Could you check a few things on this drawing? It's one solid part, dimensions in mm from its lowest x, y, z. A direction names the side the tool comes from. Round coordinates to 2 decimals unless told otherwise and drop trailing zeros. Write each loop counter-clockwise with the first axis right and the second up, starting at its lowest first coordinate (ties: lowest second). Pieces come first, ordered by that corner, then holes. Notation, with made-up numbers: (-34.5, 80.5) -> (14.5, 80.5) arc R15 cw to (14.5, 96.5) -> close; hole circle Ø6 at (39.25, -39.75). An arc over 180 degrees is marked (long way). Answer in a Markdown table with one row per item.
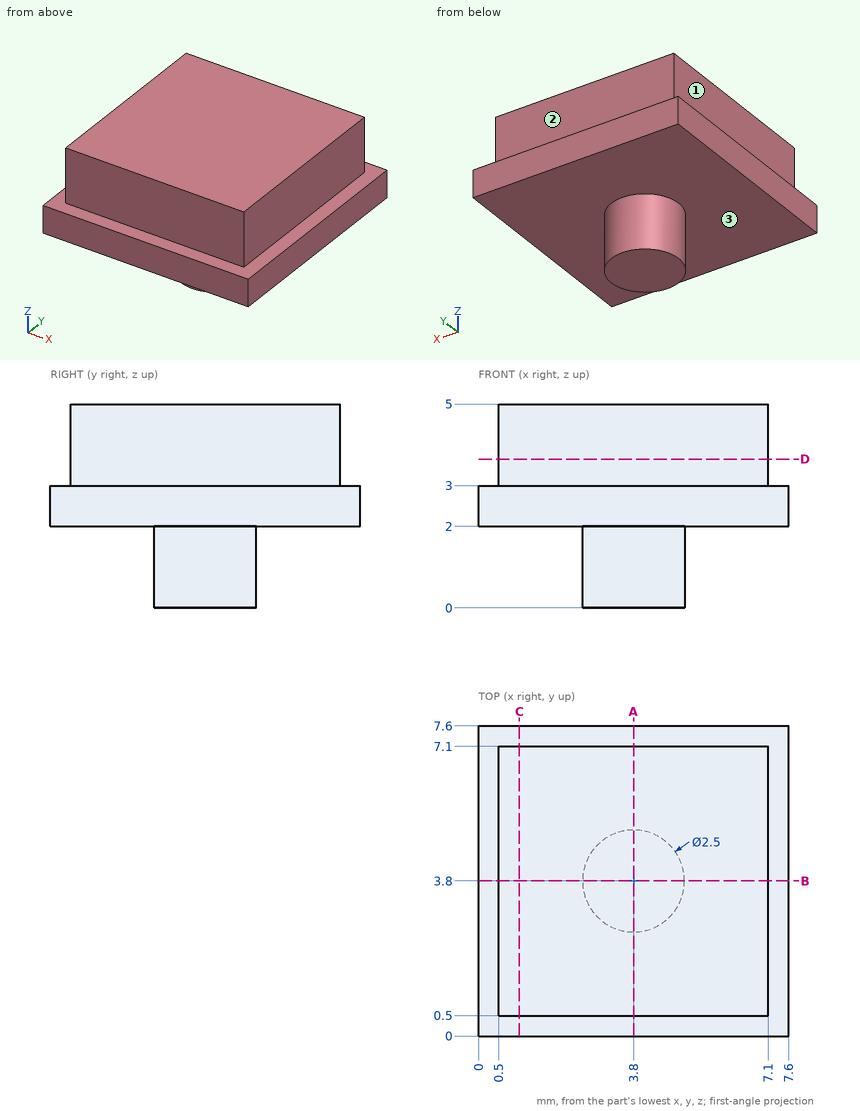
1) For pin 1 (1.6 mm diameter, centred on y = 2.5, z = 4, fed in from +X); pin 2 (3 mm diameter, centred on x = 1.5, z = 1.5, fed in from +Y); pin 3 (1 mm diameter, centred on x = 4, z = 4, fed in from -Y); pin 4 (1 mm diameter, centred on x = 4.5, y = 6.5, fed in from -Z), each with a flat end and sliding along its axis, tell me the tip position at first contact or that it passes through.
Findings:
| item | result |
|---|---|
| pin 1 | stops at x = 7.1 |
| pin 2 | stops at y = 7.6 |
| pin 3 | stops at y = 0.5 |
| pin 4 | stops at z = 2 |
2) Imagine slicing it at C-C, the plane x = 1. Please give me the cut outline in (y, z), plus the area to 3 significant figures.
Findings:
| item | result |
|---|---|
| outline | (0, 2) -> (7.6, 2) -> (7.6, 3) -> (7.1, 3) -> (7.1, 5) -> (0.5, 5) -> (0.5, 3) -> (0, 3) -> close |
| area | 20.8 mm^2 |
3) Imagine slicing it at A-A, the plane x = 3.8. Please give me the cut outline in (y, z).
Findings:
| item | result |
|---|---|
| outline | (0, 2) -> (2.55, 2) -> (2.55, 0) -> (5.05, 0) -> (5.05, 2) -> (7.6, 2) -> (7.6, 3) -> (7.1, 3) -> (7.1, 5) -> (0.5, 5) -> (0.5, 3) -> (0, 3) -> close |
4) For the marked faces 1, 2 and 3, which set-ups out of +Z, -Z, +X, -X, +Y, -Y let a thin tool reach every point of the face, with its end or its side?
Findings:
| item | result |
|---|---|
| face 1 | +Z, -X, +Y, -Y |
| face 2 | +Z, +X, -X, +Y |
| face 3 | -Z |
5) Please list where these lines run through material, in increasing order: line 1 (X direction, y = 7, z = 3.4); line 2 (Z direction, x = 2.5, y = 5.5).
Findings:
| item | result |
|---|---|
| line 1 | x = 0.5 to 7.1 |
| line 2 | z = 2 to 5 |
6) Imagine slicing it at D-D, the plane z = 3.65. Please give me the cut outline in (x, y).
Findings:
| item | result |
|---|---|
| outline | (0.5, 0.5) -> (7.1, 0.5) -> (7.1, 7.1) -> (0.5, 7.1) -> close |
